```python
from build123d import *

# Parameters (mm, degrees)
SKETCH1_W                      = 9.525
SKETCH1_H                      = 25.4
BOSS_EXTRUDE1_DEPTH            = 230.1875
CUT_EXTRUDE1_REACH             = 232.734
SKETCH2_R                      = 6.35
F_3_8_0_375_DIAMETER_HOLE1_D   = 9.525
F_8_32_TAPPED_HOLE1_AT_2_COUNT = 2
F_8_32_TAPPED_HOLE1_AT_2_PITCH = 177.8
F_8_32_TAPPED_HOLE1_AT_3_COUNT = 2
F_8_32_TAPPED_HOLE1_AT_3_PITCH = 254
F_8_32_TAPPED_HOLE1_AT_4_COUNT = 2
F_8_32_TAPPED_HOLE1_AT_4_PITCH = 431.8
F_8_32_TAPPED_HOLE1_AT_5_COUNT = 2
F_8_32_TAPPED_HOLE1_AT_5_PITCH = 342.9
F_8_32_TAPPED_HOLE1_AT_6_COUNT = 2
F_8_32_TAPPED_HOLE1_AT_6_PITCH = 88.9


with BuildPart() as part:
    # Sketch1 → Boss-Extrude1 (new, symmetric)
    with BuildSketch(Plane.XY):
        Rectangle(SKETCH1_W, SKETCH1_H)
    extrude(amount=BOSS_EXTRUDE1_DEPTH, both=True)

    # Sketch2 → Cut-Extrude1 (cut, up to next)
    with BuildSketch(Plane(origin=(4.7625, 0, 0), x_dir=(0, 0, -1), z_dir=(1, 0, 0)), mode=Mode.PRIVATE) as cut_extrude1_sk1:
        with Locations(Location((-107.95, -1.5875, 0), (0, 0, 90))):
            Circle(SKETCH2_R)
    cut_extrude1_tool1 = extrude(cut_extrude1_sk1.sketch, amount=-CUT_EXTRUDE1_REACH, mode=Mode.PRIVATE) & part.part
    # Sketch2 → Cut-Extrude1 (cut, up to next)
    with BuildSketch(Plane(origin=(4.7625, 0, 0), x_dir=(0, 0, -1), z_dir=(1, 0, 0)), mode=Mode.PRIVATE) as cut_extrude1_sk2:
        with Locations(Location((57.15, -1.5875, 0), (0, 0, 90))):
            Circle(SKETCH2_R)
    cut_extrude1_tool2 = extrude(cut_extrude1_sk2.sketch, amount=-CUT_EXTRUDE1_REACH, mode=Mode.PRIVATE) & part.part
    add(cut_extrude1_tool1.solids().sort_by_distance((4.7625, -1.5875, 107.95))[0], mode=Mode.SUBTRACT)
    add(cut_extrude1_tool2.solids().sort_by_distance((4.7625, -1.5875, -57.15))[0], mode=Mode.SUBTRACT)

    # 3/8 (0.375) Diameter Hole1 (through all)
    with Locations(Plane.ZY.offset(4.7625)):
        with Locations((85.725, -1.5875), (-85.725, -1.5875)):
            Hole(F_3_8_0_375_DIAMETER_HOLE1_D / 2)

    # Sketch5 → #8-32 Tapped Hole1 (revolve, cut)
    with BuildSketch(Plane(origin=(4.7625, -1.5875, -215.9), x_dir=(0, 0, -1), z_dir=(0, 1, 0))):
        Polygon((0, 0), (0, 9.525), (2.286, 9.525), (1.7272, 8.9662), (1.7272, 1.4478), (3.175, 0), align=None)
    f_8_32_tapped_hole1 = revolve(axis=Axis((11.1125, -1.5875, -215.9), (-1, 0, 0)), mode=Mode.SUBTRACT)

    # #8-32 Tapped Hole1 at 2: #8-32 Tapped Hole1 ×2
    with Locations(*[(0, 0, i * F_8_32_TAPPED_HOLE1_AT_2_PITCH) for i in range(1, F_8_32_TAPPED_HOLE1_AT_2_COUNT)]):
        add(f_8_32_tapped_hole1, mode=Mode.SUBTRACT)

    # #8-32 Tapped Hole1 at 3: #8-32 Tapped Hole1 ×2
    with Locations(*[(0, 0, i * F_8_32_TAPPED_HOLE1_AT_3_PITCH) for i in range(1, F_8_32_TAPPED_HOLE1_AT_3_COUNT)]):
        add(f_8_32_tapped_hole1, mode=Mode.SUBTRACT)

    # #8-32 Tapped Hole1 at 4: #8-32 Tapped Hole1 ×2
    with Locations(*[(0, 0, i * F_8_32_TAPPED_HOLE1_AT_4_PITCH) for i in range(1, F_8_32_TAPPED_HOLE1_AT_4_COUNT)]):
        add(f_8_32_tapped_hole1, mode=Mode.SUBTRACT)

    # #8-32 Tapped Hole1 at 5: #8-32 Tapped Hole1 ×2
    with Locations(*[(0, 0, i * F_8_32_TAPPED_HOLE1_AT_5_PITCH) for i in range(1, F_8_32_TAPPED_HOLE1_AT_5_COUNT)]):
        add(f_8_32_tapped_hole1, mode=Mode.SUBTRACT)

    # #8-32 Tapped Hole1 at 6: #8-32 Tapped Hole1 ×2
    with Locations(*[(0, 0, i * F_8_32_TAPPED_HOLE1_AT_6_PITCH) for i in range(1, F_8_32_TAPPED_HOLE1_AT_6_COUNT)]):
        add(f_8_32_tapped_hole1, mode=Mode.SUBTRACT)


solid = part.part
```
Verification items for the finished model (mm, model axes). Round coordinates to 2 decimals unless told otherwise and drop trailing zeros. Order: outer loops, then holes, each group sorted by start corner. A loop starts at its lowest first (then second) coordinate and runs counter-clockwise, first axis right, second up. Notation, with made-up numbers: (64.5, 74.5) - (73.5, 74.5) arc R30 ccw to (73.5, 109.5) - close; hole circle Ø8 at (41.25, -32.75). An arc over 180 degrees is marked (long way). Use CSV: the item, a comma, the result in double quotes.
(1) Gauge pin test, flat ends, axial feed: pin 1 Ø5.5 at (y, z) = (-1.59, -127) entering from +X; pin 2 Ø4 at (y, z) = (-1.59, 215.9) entering from +X; pin 3 Ø2 at (y, z) = (-3, 37) entering from +X. Record the tip position at first contact, or that the pin passes through.
Entries:
pin 1,"x = 4.34"
pin 2,"x = 3.59"
pin 3,"x = 4.38"
(2) Mould release check, pull along Z, two halves, no side actions. Record for faces 1 (the face through (0, 12.7, 3)), 2 (the face through (0, 0, -230.188)), 3 (the face through (0.07, -2.96, 101.75)): released by +Z, released by -Z, zero draft, split by the parting line, or undercut.
Entries:
face 1,"zero draft"
face 2,"released by -Z"
face 3,"undercut"
(3) Thickness scan on probe 1 along Y at (x, z) = (-0.25, -215.9); probe 2 along Z at (x, y) = (1.5, -5.5); probe 3 along Z at (x, y) = (3.5, -5.25). Record the ranges inside material, lowest first. Write a range as from..to.
Entries:
probe 1,"-12.7..-3.31, 0.14..12.7"
probe 2,"-230.19..-88.44, -83.01..-62.15, -52.15..83.01, 88.44..102.95, 112.95..230.19"
probe 3,"-230.19..-88.77, -82.68..-62.34, -51.96..82.68, 88.77..102.76, 113.14..230.19"
(4) Section check C-C on z = 86. Record the boundary of the cut face in (x, y), and give its area (3 significant figures).
Entries:
outline,"(-4.76, -12.7) - (4.76, -12.7) - (4.76, -6.34) - (-4.76, -6.34) - close; (-4.76, 3.17) - (4.76, 3.17) - (4.76, 12.7) - (-4.76, 12.7) - close"
area,"151 mm^2"
(5) Section check B-B on x = -2. State how many separate pieces and enclosed holes the cut face has, and give its area (3 significant figures).
Entries:
separate pieces,"1"
enclosed holes,"10"
area,"11,200 mm^2"
(6) Section check A-A on z = -57.15. Record the boundary of the cut face in (x, y), and give its area (3 significant figures).
Entries:
outline,"(-4.76, -12.7) - (4.76, -12.7) - (4.76, -7.94) - (-4.76, -7.94) - close; (-4.76, 4.76) - (4.76, 4.76) - (4.76, 12.7) - (-4.76, 12.7) - close"
area,"121 mm^2"
